```python
from build123d import *

# Parameters (mm, degrees)
SKETCH1_W                    = 25.4
SKETCH1_H                    = 50.8
SKETCH1_W_2                  = 19.05
SKETCH1_H_2                  = 44.45
BOSS_EXTRUDE1_DEPTH          = 101.6
CUT_EXTRUDE1_DEPTH           = 115.3
CUT_EXTRUDE2_DEPTH           = 108.763073453
SKETCH4_W                    = 34.925
SKETCH4_H                    = 34.925
CUT_EXTRUDE3_DEPTH           = 108.763073453
F_10_0_1935_DIAMETER_HOLE1_D = 4.9149
FILLET1_R                    = 6.35
F_10_0_1935_DIAMETER_HOLE2_D = 4.9149


with BuildPart() as part:
    # Sketch1 → Boss-Extrude1 (new body)
    with BuildSketch(Plane(origin=(0, 0, 0), x_dir=(1, 0, 0), z_dir=(0, 1, 0))):
        Rectangle(SKETCH1_W, SKETCH1_H)
        Rectangle(SKETCH1_W_2, SKETCH1_H_2, mode=Mode.SUBTRACT)
    extrude(amount=BOSS_EXTRUDE1_DEPTH)

    # Sketch2 → Cut-Extrude1 (cut, through all)
    with BuildSketch(Plane.XY.offset(25.4)):
        Polygon((12.7, 101.6), (-12.7, 101.6), (12.7, 94.794090512), align=None)
    extrude(amount=-CUT_EXTRUDE1_DEPTH, mode=Mode.SUBTRACT)

    # Sketch3 → Cut-Extrude2 (cut, through all)
    with BuildSketch(Plane.ZY.offset(12.7)):
        with BuildLine():
            Line((-25.4, 12.7), (-25.4, 0))
            Line((-25.4, 0), (-12.7, 0))
            ThreePointArc((-12.7, 0), (-21.680256121, 3.719743879), (-25.4, 12.7))
        make_face()
        with BuildLine():
            ThreePointArc((25.4, 12.7), (21.680256121, 3.719743879), (12.7, 0))
            Line((12.7, 0), (25.4, 0))
            Line((25.4, 0), (25.4, 12.7))
        make_face()
    extrude(amount=-CUT_EXTRUDE2_DEPTH, mode=Mode.SUBTRACT)

    # Sketch4 → Cut-Extrude3 (cut, through all)
    with BuildSketch(Plane.ZY.offset(12.7)):
        with Locations((0, 38.1)):
            Rectangle(SKETCH4_W, SKETCH4_H)
    extrude(amount=-CUT_EXTRUDE3_DEPTH, mode=Mode.SUBTRACT)

    # #10 (0.1935) Diameter Hole1 (through all)
    with Locations(Plane.ZY.offset(12.7)):
        with Locations((0, 61.9125), (0, 14.2875)):
            Hole(F_10_0_1935_DIAMETER_HOLE1_D / 2)

    # Fillet1
    fillet1_edges = [part.edges().sort_by_distance(p)[0] for p in [
        (-11.1125, 20.6375, -17.4625),
        (-11.1125, 55.5625, -17.4625),
        (-11.1125, 55.5625, 17.4625),
        (-11.1125, 20.6375, 17.4625),
        (11.1125, 20.6375, -17.4625),
        (11.1125, 55.5625, -17.4625),
        (11.1125, 55.5625, 17.4625),
        (11.1125, 20.6375, 17.4625),
    ]]
    fillet(fillet1_edges, radius=FILLET1_R)

    # #10 (0.1935) Diameter Hole2 (through all)
    with Locations(Plane.ZY.offset(12.7)):
        with Locations((-12.7, 88.9), (12.7, 88.9)):
            Hole(F_10_0_1935_DIAMETER_HOLE2_D / 2)


solid = part.part
```
Check sheet for the modelled part. Datum: model origin and axes. Units: mm. A direction names the side the tool comes from. Round coordinates to 2 decimals unless told otherwise and drop trailing zeros. Order: outer loops, then holes, each group sorted by start corner. A loop starts at its lowest first (then second) coordinate and runs counter-clockwise, first axis right, second up. Notation, with made-up numbers: M 14.25,-17 L 49.25,-17 A21 cw 49.25,3 Z; hole C -15,58 d8. An arc over 180 degrees is marked long. Answer in a Markdown table with one row per item.
(1) Section check A-A on z = -3.5. Record the boundary of the cut face in (x, y) (1 decimal), plus the area to 3 significant figures.
Findings:
| item | result |
|---|---|
| outline | M -12.7,0 L -9.5,0 L -9.5,20.6 L -12.7,20.6 Z; M -12.7,55.6 L -9.5,55.6 L -9.5,100.7 L -12.7,101.6 Z; M 9.5,0 L 12.7,0 L 12.7,20.6 L 9.5,20.6 Z; M 9.5,55.6 L 12.7,55.6 L 12.7,94.8 L 9.5,95.6 Z |
| area | 402 mm^2 |
(2) Section check B-B on x = 8.5. Record the boundary of the cut face in (y, z) (3 decimals).
Findings:
| item | result |
|---|---|
| outline | M 4.3,-22.225 A12.7 ccw 12.7,-25.4 L 95.919,-25.4 L 95.919,-22.225 Z; M 4.3,22.225 L 95.919,22.225 L 95.919,25.4 L 12.7,25.4 A12.7 ccw Z |
(3) Section check D-D on z = -19.5. Record the boundary of the cut face in (x, y) (3 decimals), plus the area to 3 significant figures.
Findings:
| item | result |
|---|---|
| outline | M -12.7,1.974 L -9.525,1.974 L -9.525,100.749 L -12.7,101.6 Z; M 9.525,1.974 L 12.7,1.974 L 12.7,94.794 L 9.525,95.645 Z |
| area | 611 mm^2 |
(4) Draft check along Y on faces 4 (the cylindrical face through (11.135, 91.337, 13.02)), 5 (the flat face through (11, 0, 0)), 6 (the flat face through (9.525, 58, 0)). Enter one of: +Y half, -Y half, draft (parallel to the pull), parting line (faces both ways), or undercut.
Findings:
| item | result |
|---|---|
| face 4 | undercut |
| face 5 | -Y half |
| face 6 | draft |
(5) Section check C-C on y = 65.5. Record the boundary of the cut face in (x, z) (3 decimals), plus the area to 3 significant figures.
Findings:
| item | result |
|---|---|
| outline | M -12.7,-25.4 L 12.7,-25.4 L 12.7,25.4 L -12.7,25.4 Z; hole M -9.525,-22.225 L 9.525,-22.225 L 9.525,22.225 L -9.525,22.225 Z |
| area | 444 mm^2 |
(6) Set-up check for faces 1 (the flat face through (-9.525, 61, 5)), 2 (the flat face through (-11, 20.638, 0)), 3 (the cylindrical face through (-0.18, 7.46, 24.27)): record each of +Z, -Z, +X, -X, +Y, -Y from which the full face is reachable in a straight line by a thin tool's end or side.
Findings:
| item | result |
|---|---|
| face 1 | +Y, -Y |
| face 2 | +X, -X |
| face 3 | +Z, +X, -X, -Y |
(7) Gauge pin test, flat ends, axial feed: pin 1 (1 mm diameter, centred on x = 10.5, z = -2.5, fed in from +Y); pin 2 (8 mm diameter, centred on y = 88.9, z = 12.7, fed in from -X); pin 3 (3 mm diameter, centred on x = 10, z = -9.5, fed in from +Y). Record the tip position at first contact, or that the pin passes through.
Findings:
| item | result |
|---|---|
| pin 1 | stops at y = 95.52 |
| pin 2 | stops at x = -12.7 |
| pin 3 | stops at y = 95.64 |
(8) Material ranges on line 1 along X through (y, z) = (56.5, -11.5) (3 decimals); line 2 along Z through (x, y) = (1.75, 54.5) (3 decimals); line 3 along Y through (x, z) = (11.85, 0), recorded low to high. Write a range as from..to.
Findings:
| item | result |
|---|---|
| line 1 | x = -12.7..-9.525, 9.525..12.7 |
| line 2 | z = -25.4..-22.225, 22.225..25.4 |
| line 3 | y = 0..11.83, 16.74..20.64, 55.56..59.46, 64.37..95.02 |
